```python
from build123d import *

# Parameters (mm, degrees)
F0_W      = 180
F0_H      = 150
F1_DEPTH  = 50
F2_T      = -2.5
F3_W      = 20.1315768063
F3_H      = 50
F4_DEPTH  = 25
F5_W      = 20.1315768063
F5_H      = 50
F6_DEPTH  = 25
F7_W      = 20.131578669
F7_H      = 50
F8_DEPTH  = 25
F9_W      = 6.2171062455
F9_H      = 50
F10_DEPTH = 25


with BuildPart() as f1:
    # F0 (on Top) → F1 (new body)
    with BuildSketch(Plane.XY):
        Rectangle(F0_W, F0_H)
    extrude(amount=F1_DEPTH)

    # F2
    f2_openings = [f1.faces().sort_by_distance(p)[0] for p in [
        (0, 0, 50),
    ]]
    offset(amount=F2_T, openings=f2_openings)

    # F3 (on face) → F4 (cut)
    with BuildSketch(Plane.XZ.offset(75)):
        with Locations((-64.5394753665, 25)):
            Rectangle(F3_W, F3_H)
    extrude(amount=-F4_DEPTH, mode=Mode.SUBTRACT)

    # F5 (on face) → F6 (cut)
    with BuildSketch(Plane.XZ.offset(75)):
        with Locations((-29.9013163894, 25)):
            Rectangle(F5_W, F5_H)
    extrude(amount=-F6_DEPTH, mode=Mode.SUBTRACT)

    # F7 (on face) → F8 (cut)
    with BuildSketch(Plane.XZ.offset(75)):
        with Locations((10.0657893345, 25)):
            Rectangle(F7_W, F7_H)
    extrude(amount=-F8_DEPTH, mode=Mode.SUBTRACT)

    # F9 (on face) → F10 (cut)
    with BuildSketch(Plane.XZ.offset(75)):
        with Locations((-16.7269748636, 25)):
            Rectangle(F9_W, F9_H)
    extrude(amount=-F10_DEPTH, mode=Mode.SUBTRACT)


solid = f1.part
```
Geometry: final body of the model. Coordinates: model frame, mm. A direction names the side the tool comes from. Coordinates: 2 decimals unless noted, no trailing zeros. Write each loop counter-clockwise with the first axis right and the second up, starting at its lowest first coordinate (ties: lowest second). Pieces come first, ordered by that corner, then holes. Notation, with made-up numbers: M 43.25,-33 L 90.25,-33 A19 cw 90.25,-29 Z; hole C 52.5,59.25 d8. An arc over 180 degrees is marked long. Use CSV: the item, a comma, the result in double quotes. Start each with the question number.
1. Cut plane D-D on y = 11.5. Return the cut outline in (x, z), plus the area to 4 significant figures.
2. First-contact query: P1, Ø1.2, axis at x = -65, z = 1.5, coming from the -Y side; P2, Ø3, axis at x = 5.5, y = -28, coming from the +Z side; P3, Ø4, axis at x = 5.5, z = 36.5, coming from the -Y side. Flat tips, straight axial feed; report the tip coordinate or a pass-through.
3. Cut plane A-A on z = 36. Return the cut outline in (x, y).
4. Cut plane B-B on y = -61.5. Return the cut outline in (x, z).
5. Mould query, pull axis Y, two halves, no side actions, for faces 1 (the face through (-47, -75, 25)), 2 (the face through (87.5, -1, 26)), 3 (the face through (-54.474, -73, 19)), 4 (the face through (-1, 72.5, 26)). Classes: pulls with the +Y half, pulls with the -Y half, needs draft (parallel to the pull), parting line crosses it, or undercut.
6. Cut plane C-C on x = 29. Return the cut outline in (y, z), plus the area to 4 significant figures.
7. Ray query, probe 1 along Y at (x, z) = (74.5, 19); probe 2 along X at (y, z) = (0, 22.5); probe 3 along Z at (x, y) = (57.5, 41.5). Return the intervals inside material, ascending.
8. Reachability of faces 5 (the face through (-1, 1, 2.5)), 6 (the face through (-39.967, -73, 19)), 7 (the face through (0, 73, 50)) from +Z, -Z, +X, -X, +Y, -Y: full face, straight path, thin tool, end or side. Return the list, or none.
Entries:
1,outline,"M -90,0 L 90,0 L 90,50 L 87.5,50 L 87.5,2.5 L -87.5,2.5 L -87.5,50 L -90,50 Z"
1,area,"687.5 mm²"
2,P1,"y = -50"
2,P2,"z = 2.5"
2,P3,"y = 72.5"
3,outline,"M -90,-75 L -74.61,-75 L -74.61,-72.5 L -87.5,-72.5 L -87.5,72.5 L 87.5,72.5 L 87.5,-72.5 L 20.13,-72.5 L 20.13,-75 L 90,-75 L 90,75 L -90,75 Z; M -54.47,-75 L -39.97,-75 L -39.97,-72.5 L -54.47,-72.5 Z; M -13.62,-75 L 0,-75 L 0,-72.5 L -13.62,-72.5 Z"
4,outline,"M -90,0 L -74.61,0 L -74.61,2.5 L -87.5,2.5 L -87.5,50 L -90,50 Z; M -54.47,0 L -39.97,0 L -39.97,2.5 L -54.47,2.5 Z; M -13.62,0 L 0,0 L 0,2.5 L -13.62,2.5 Z; M 20.13,0 L 90,0 L 90,50 L 87.5,50 L 87.5,2.5 L 20.13,2.5 Z"
5,face 1,"pulls with the -Y half"
5,face 2,"undercut"
5,face 3,"needs draft"
5,face 4,"undercut"
6,outline,"M -75,0 L 75,0 L 75,50 L 72.5,50 L 72.5,2.5 L -72.5,2.5 L -72.5,50 L -75,50 Z"
6,area,"612.5 mm²"
7,probe 1,"-75 to -72.5, 72.5 to 75"
7,probe 2,"-90 to -87.5, 87.5 to 90"
7,probe 3,"0 to 2.5"
8,face 5,"+Z"
8,face 6,"+Z, -Z, -Y"
8,face 7,"+Z, +X, -X, +Y, -Y"
